from build123d import *

# Parameters (mm, degrees)
SKETCH1_W           = 90
SKETCH1_H           = 60
BOSS_EXTRUDE1_DEPTH = 1.6
FILLET1_R           = 5
SKETCH2_R           = 1.5
CUT_EXTRUDE1_DEPTH  = 1.6


with BuildPart() as part:
    # Sketch1 → Boss-Extrude1 (new body)
    with BuildSketch(Plane.XY):
        with Locations((45, 30)):
            Rectangle(SKETCH1_W, SKETCH1_H)
    extrude(amount=BOSS_EXTRUDE1_DEPTH)

    # Fillet1
    fillet1_edges = [part.edges().sort_by_distance(p)[0] for p in [
        (0, 60, 0.8),
        (90, 60, 0.8),
        (90, 0, 0.8),
        (0, 0, 0.8),
    ]]
    fillet(fillet1_edges, radius=FILLET1_R)

    # Sketch2 → Cut-Extrude1 (cut)
    with BuildSketch(Plane.XY.offset(1.6)):
        with Locations((79, 56)):
            Circle(SKETCH2_R)
        with Locations((3, 56)):
            Circle(SKETCH2_R)
    cut_extrude1 = extrude(amount=-CUT_EXTRUDE1_DEPTH, mode=Mode.SUBTRACT)

    # Mirror1: Cut-Extrude1 across plane
    add(cut_extrude1.mirror(Plane(origin=(0, 30, 0), x_dir=(0, 0, 1), z_dir=(0, -1, 0))), mode=Mode.SUBTRACT)


solid = part.part
Check sheet for the modelled part. Datum: model origin and axes. Units: mm. Give positions to 0.01 mm unless a question says otherwise; leave off trailing zeros. Write each loop counter-clockwise with the first axis right and the second up, starting at its lowest first coordinate (ties: lowest second). Pieces come first, ordered by that corner, then holes. Notation, with made-up numbers: (77, 64) -> (111, 64) arc R13 cw to (111, 70) -> close; hole circle Ø5 at (-29.75, 14). An arc over 180 degrees is marked (long way). Write item = value, one per line.
Item 1: Sectioned sample at B-B on y = 56. Record the boundary of the cut face in (x, z), and give its area (3 significant figures).
Output:
outline = (0.1, 0) -> (1.5, 0) -> (1.5, 1.6) -> (0.1, 1.6) -> close; (4.5, 0) -> (77.5, 0) -> (77.5, 1.6) -> (4.5, 1.6) -> close; (80.5, 0) -> (89.9, 0) -> (89.9, 1.6) -> (80.5, 1.6) -> close
area = 134 mm^2
Item 2: Release check for a two-part mould opening along Y. For faces 1 (the cylindrical face through (88, 1, 1)), 2 (the cylindrical face through (80.43, 56.45, 0.81)), 3 (the flat face through (44, 30, 1.6)) record: +Y half, -Y half, draft (parallel to the pull), parting line (faces both ways), or undercut.
Output:
face_1 = -Y half
face_2 = undercut
face_3 = draft
Item 3: Gauge pin test, flat ends, axial feed: pin 1 (10 mm diameter, centred on x = 67.5, y = 35.5, fed in from -Z); pin 2 (1.8 mm diameter, centred on x = 79, y = 4, fed in from -Z). Record the tip position at first contact, or that the pin passes through.
Output:
pin_1 = 0
pin_2 = through
Item 4: Scan lines: probe 1 along Y at (x, z) = (79, 0.95); probe 2 along X at (y, z) = (5, 0.6); probe 3 along X at (y, z) = (4, 1.05). Record each from-to range of solid material in increasing order. Write a range as from..to.
Output:
probe_1 = 0..2.5, 5.5..54.5, 57.5..60
probe_2 = 0..1.88, 4.12..77.88, 80.12..90
probe_3 = 0.1..1.5, 4.5..77.5, 80.5..89.9
Item 5: Sectioned sample at A-A on x = 79. Record the boundary of the cut face in (y, z).
Output:
outline = (0, 0) -> (2.5, 0) -> (2.5, 1.6) -> (0, 1.6) -> close; (5.5, 0) -> (54.5, 0) -> (54.5, 1.6) -> (5.5, 1.6) -> close; (57.5, 0) -> (60, 0) -> (60, 1.6) -> (57.5, 1.6) -> close
